from build123d import *

# Parameters (mm, degrees)
SKETCH1_R           = 11.43
BOSS_EXTRUDE2_DEPTH = 12.7


with BuildPart() as part:
    # Sketch1 → Boss-Extrude2 (new body)
    with BuildSketch(Plane.XY):
        with BuildLine():
            Line((103.972822377, 346.773604775), (173.822822377, 346.773604775))
            Line((173.822822377, 346.773604775), (173.822822377, 35.623604775))
            Line((173.822822377, 35.623604775), (173.822822377, 29.273604775))
            Line((173.822822377, 29.273604775), (161.122822377, 29.273604775))
            Line((161.122822377, 29.273604775), (151.597822377, 29.273604775))
            ThreePointArc((151.597822377, 29.273604775), (147.107694316, 31.133476714), (145.247822377, 35.623604775))
            Line((145.247822377, 35.623604775), (145.247822377, 61.023604775))
            ThreePointArc((145.247822377, 61.023604775), (143.387950437, 65.513732836), (138.897822377, 67.373604775))
            Line((138.897822377, 67.373604775), (30.947822377, 67.373604775))
            ThreePointArc((30.947822377, 67.373604775), (26.457694316, 65.513732836), (24.597822377, 61.023604775))
            Line((24.597822377, 61.023604775), (24.597822377, 35.623604775))
            ThreePointArc((24.597822377, 35.623604775), (22.737950437, 31.133476714), (18.247822377, 29.273604775))
            Line((18.247822377, 29.273604775), (2.372822377, 29.273604775))
            Line((2.372822377, 29.273604775), (-3.977177623, 29.273604775))
            Line((-3.977177623, 29.273604775), (-3.977177623, 35.623604775))
            Line((-3.977177623, 35.623604775), (-3.977177623, 346.773604775))
            Line((-3.977177623, 346.773604775), (65.872822377, 346.773604775))
            Line((65.872822377, 346.773604775), (65.872822377, 302.323604775))
            ThreePointArc((65.872822377, 302.323604775), (67.732694316, 297.833476714), (72.222822377, 295.973604775))
            Line((72.222822377, 295.973604775), (97.622822377, 295.973604775))
            ThreePointArc((97.622822377, 295.973604775), (102.112950437, 297.833476714), (103.972822377, 302.323604775))
            Line((103.972822377, 302.323604775), (103.972822377, 346.773604775))
        make_face()
        with Locations((34.122822377, 295.973604775)):
            Circle(SKETCH1_R, mode=Mode.SUBTRACT)
    extrude(amount=BOSS_EXTRUDE2_DEPTH)


solid = part.part
Verification items for the finished model (mm, model axes). A direction names the side the tool comes from. Round coordinates to 2 decimals unless told otherwise and drop trailing zeros. Loops run counter-clockwise (first coordinate to the right, second up) from the corner with the lowest first, then second, coordinate; pieces in that order, holes last. Notation, with made-up numbers: (37, 7) - (79, 7) arc R21 cw to (79, 15) - close; hole circle Ø9 at (9.25, 56.5). An arc over 180 degrees is marked (long way). Use a Markdown table: item, result. Add a question column.
1. Access from +Z, -Z, +X, -X, +Y, -Y to the whole of each face (thin tool, end or side, straight path). Record for faces 1 (the face through (163, 29.274, 6)), 2 (the face through (102.06, 297.78, 6.26)), 3 (the face through (86, 67.374, 6)).
2. Thickness scan on probe 1 along X at (y, z) = (52.5, 11); probe 2 along Y at (x, z) = (35, 1); probe 3 along Y at (x, z) = (116, 6.25). Record the ranges inside material, lowest first. Write a range as [from, to].
3. Gauge pin test, flat ends, axial feed: pin 1 (2 mm diameter, centred on x = 56, z = 5, fed in from -Y); pin 2 (1.5 mm diameter, centred on x = 155, y = 277.5, fed in from -Z). Record the tip position at first contact, or that the pin passes through.
4. Section check A-A, the plane y = 318. Record the boundary of the cut face in (x, z).
5. Section check C-C, the plane x = 58. Record the boundary of the cut face in (y, z), plus the area to 3 significant figures.
6. Release check for a two-part mould opening along Y. For faces 4 (the face through (138, 346.774, 6)), 5 (the face through (32.6, 307.3, 6.3)), 6 (the face through (145.248, 48, 6)) record: released by +Y, released by -Y, zero draft, split by the parting line, or undercut.
7. Section check B-B, the plane z = 6.25. Record the boundary of the cut face in (x, y), plus the area to 3 significant figures.
Checks:
| question | item | result |
|---|---|---|
| 1 | face 1 | +Z, -Z, +X, -X, -Y |
| 1 | face 2 | +Z, -Z, +Y |
| 1 | face 3 | +Z, -Z, -Y |
| 2 | probe 1 | x = [-3.98, 24.6], [145.25, 173.82] |
| 2 | probe 2 | y = [67.37, 284.58], [307.37, 346.77] |
| 2 | probe 3 | y = [67.37, 346.77] |
| 3 | pin 1 | stops at y = 67.37 |
| 3 | pin 2 | stops at z = 0 |
| 4 | outline | (-3.98, 0) - (65.87, 0) - (65.87, 12.7) - (-3.98, 12.7) - close; (103.97, 0) - (173.82, 0) - (173.82, 12.7) - (103.97, 12.7) - close |
| 5 | outline | (67.37, 0) - (346.77, 0) - (346.77, 12.7) - (67.37, 12.7) - close |
| 5 | area | 3,550 mm^2 |
| 6 | face 4 | released by +Y |
| 6 | face 5 | undercut |
| 6 | face 6 | zero draft |
| 7 | outline | (-3.98, 29.27) - (18.25, 29.27) arc R6.35 ccw to (24.6, 35.62) - (24.6, 61.02) arc R6.35 cw to (30.95, 67.37) - (138.9, 67.37) arc R6.35 cw to (145.25, 61.02) - (145.25, 35.62) arc R6.35 ccw to (151.6, 29.27) - (173.82, 29.27) - (173.82, 346.77) - (103.97, 346.77) - (103.97, 302.32) arc R6.35 cw to (97.62, 295.97) - (72.22, 295.97) arc R6.35 cw to (65.87, 302.32) - (65.87, 346.77) - (-3.98, 346.77) - close; hole circle Ø22.86 at (34.12, 295.97) |
| 7 | area | 49,500 mm^2 |
